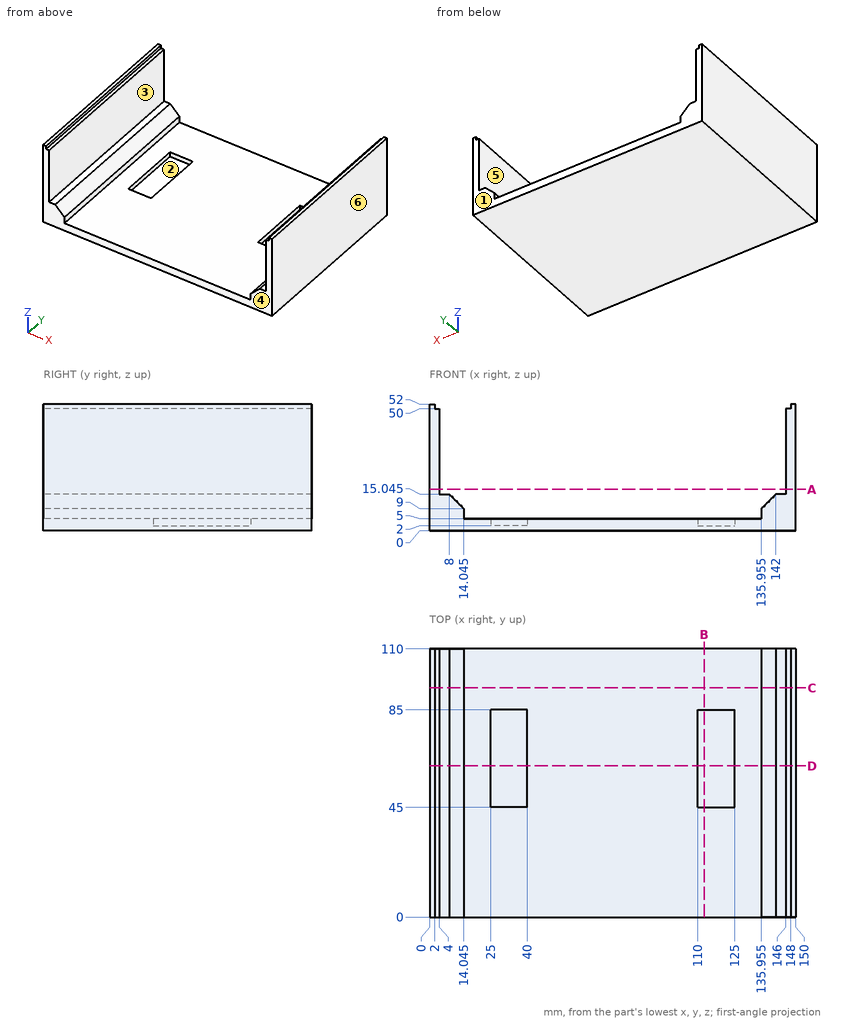
The drawing under review shows one solid part. Ordinate dimensions are in mm from its lowest x, y, z. A direction names the side the tool comes from. Round coordinates to 2 decimals unless told otherwise and drop trailing zeros. Loops run counter-clockwise (first coordinate to the right, second up) from the corner with the lowest first, then second, coordinate; pieces in that order, holes last. Notation, with made-up numbers: (21, -7.75) - (67, -7.75) arc R21 cw to (67, 11.25) - close; hole circle Ø2 at (70, -2). An arc over 180 degrees is marked (long way). Put each result on its own line as item: value. Start each with the question number.
1. Mouldability with a two-part tool opening along X and no side actions: class the marked faces 4, 5 and 6 as +X half, -X half, draft (parallel to the pull), parting line (faces both ways), or undercut.
2. Consider section B-B on x = 112.5. State the section outline as (y, z) points, plus the area to 3 significant figures.
3. For probe 1 along X at (y, z) = (24.5, 22); probe 2 along Z at (x, y) = (142, 36) (1 decimal); probe 3 along Z at (x, y) = (21, 88.5), list the stretches that pass through material, from the lowest coordinate up. Write a range as [from, to].
4. Consider section C-C on y = 94. State the section outline as (x, z) points (1 decimal).
5. For the marked faces 1, 2 and 3, list the 3-axis set-ups (+Z, -Z, +X, -X, +Y, -Y) from which the entire face can be reached by the end or side of a thin tool; tool diameter is ignored.
6. Consider section A-A on z = 17. State the section outline as (x, y) points.
7. Insertion check: P1, Ø16.5, axis at x = 36, y = 59, coming from the +Z side; P2, Ø1, axis at x = 147, y = 53.5, coming from the +Z side; P3, Ø2, axis at x = 144, y = 60, coming from the +Z side (1 decimal). Each pin has a flat end and moves straight along its axis. Give the tip position at first contact, or say it passes through.
8. Consider section D-D on y = 62. State the section outline as (x, z) points (1 decimal), plus the area to 3 significant figures.
Result sheet:
1. face 4: draft
1. face 5: undercut
1. face 6: +X half
2. outline: (0, 0) - (110, 0) - (110, 5) - (85, 5) - (85, 2) - (45, 2) - (45, 5) - (0, 5) - close
2. area: 430 mm^2
3. probe 1: [0, 4], [146, 150]
3. probe 2: [0, 15]
3. probe 3: [0, 5]
4. outline: (0, 0) - (150, 0) - (150, 52) - (148, 52) - (148, 50) - (146, 50) - (146, 15) - (142, 15) - (136, 9) - (136, 5) - (14, 5) - (14, 9) - (8, 15) - (4, 15) - (4, 50) - (2, 50) - (2, 52) - (0, 52) - close
5. face 1: +Z, -Z, +X, -X, +Y
5. face 2: +Z
5. face 3: +Z, +Y, -Y
6. outline: (0, 0) - (4, 0) - (4, 110) - (0, 110) - close; (146, 0) - (150, 0) - (150, 110) - (146, 110) - close
7. P1: z = 5
7. P2: z = 50
7. P3: z = 15
8. outline: (0, 0) - (150, 0) - (150, 52) - (148, 52) - (148, 50) - (146, 50) - (146, 15) - (142, 15) - (136, 9) - (136, 5) - (125, 5) - (125, 2) - (110, 2) - (110, 5) - (40, 5) - (40, 2) - (25, 2) - (25, 5) - (14, 5) - (14, 9) - (8, 15) - (4, 15) - (4, 50) - (2, 50) - (2, 52) - (0, 52) - close
8. area: 1,190 mm^2
